from build123d import *

# Parameters (mm, degrees)
ESQUISSE1_W        = 10
ESQUISSE1_H        = 30
ESQUISSE1_R        = 1.55
BOSS_EXTRU_1_DEPTH = 3
ESQUISSE3_W        = 10
ESQUISSE3_H        = 10
ESQUISSE3_R        = 1.4
BOSS_EXTRU_2_DEPTH = 3
CONG_1_R           = 2


with BuildPart() as part:
    # Esquisse1 → Boss.-Extru.1 (new body)
    with BuildSketch(Plane.XY):
        Rectangle(ESQUISSE1_W, ESQUISSE1_H)
        with Locations((0, 12)):
            Circle(ESQUISSE1_R, mode=Mode.SUBTRACT)
        with Locations((0, -12.5)):
            Circle(ESQUISSE1_R, mode=Mode.SUBTRACT)
    extrude(amount=BOSS_EXTRU_1_DEPTH)

    # Esquisse3 → Boss.-Extru.2 (add)
    with BuildSketch(Plane.XY.offset(3)):
        with Locations((0, -20)):
            Rectangle(ESQUISSE3_W, ESQUISSE3_H)
        with Locations((0, -22)):
            Circle(ESQUISSE3_R, mode=Mode.SUBTRACT)
    extrude(amount=-BOSS_EXTRU_2_DEPTH)

    # Congé1
    cong_1_edges = [part.edges().sort_by_distance(p)[0] for p in [
        (-5, -25, 1.5),
        (5, -25, 1.5),
        (-5, 15, 1.5),
        (5, 15, 1.5),
    ]]
    fillet(cong_1_edges, radius=CONG_1_R)


solid = part.part
Here's how the part is built. I have some questions about the finished solid (model axes, mm). Round coordinates to 2 decimals unless told otherwise and drop trailing zeros. Loops run counter-clockwise (first coordinate to the right, second up) from the corner with the lowest first, then second, coordinate; pieces in that order, holes last. Notation, with made-up numbers: M -13,-35 L -3,-35 A11 ccw -3,-26 Z; hole C 24.25,75.25 d7. An arc over 180 degrees is marked long. Write each question's results on one line, items separated by ' | '. Start each with the question number.
(1) I want a section at C-C (y = -12.5). Please give me the cut outline in (x, z), then the cut area to 3 significant figures.
(2) Thinking about a two-plate mould opening in X: for faces 1 (the flat face through (0, -5, 3)), 2 (the cylindrical face through (-0.303, -23.367, 1.521)), 3 (the cylindrical face through (4.43, 14.4, 1.52)), which applies, pulls with the +X half, pulls with the -X half, needs draft (parallel to the pull), parting line crosses it, or undercut?
(3) Will this pin go through, and if not, where does the flat tip stop? P1, Ø1, axis at x = -4, z = 1.5, coming from the +Y side.
(4) I want a section at A-A (x = 0). Please give me the cut outline in (y, z), then the cut area to 3 significant figures.
(5) I want a section at B-B (z = 0.4). Please give me the cut outline in (x, y).
(6) If I drill on probe 1 along Y at (x, z) = (0, 0.7); probe 2 along Y at (x, z) = (-0.75, 1.3); probe 3 along Y at (x, z) = (-3.5, 1.15), over which ranges is the centre line in solid material (lowest first)? Write a range as from..to.
Solved:
1) outline: M -5,0 L -1.55,0 L -1.55,3 L -5,3 Z; M 1.55,0 L 5,0 L 5,3 L 1.55,3 Z | area: 20.7 mm²
2) face 1: needs draft | face 2: undercut | face 3: pulls with the +X half
3) P1: stops at y = 14.94
4) outline: M -25,0 L -23.4,0 L -23.4,3 L -25,3 Z; M -20.6,0 L -14.05,0 L -14.05,3 L -20.6,3 Z; M -10.95,0 L 10.45,0 L 10.45,3 L -10.95,3 Z; M 13.55,0 L 15,0 L 15,3 L 13.55,3 Z | area: 93.0 mm²
5) outline: M -5,-23 A2 ccw -3,-25 L 3,-25 A2 ccw 5,-23 L 5,13 A2 ccw 3,15 L -3,15 A2 ccw -5,13 Z; hole C 0,-12.5 d3.1; hole C 0,12 d3.1; hole C 0,-22 d2.8
6) probe 1: y = -25..-23.4, -20.6..-14.05, -10.95..10.45, 13.55..15 | probe 2: y = -25..-23.18, -20.82..-13.86, -11.14..10.64, 13.36..15 | probe 3: y = -24.94..14.94
